```python
from build123d import *

# Parameters (mm, degrees)
SKETCH_1_R      = 1.35
SKETCH_1_R_2    = 1.3
EXTRUDE_1_DEPTH = 3


with BuildPart() as part:
    # 草图1 → 凸台-拉伸1 (new body)
    with BuildSketch(Plane.XY.offset(3)):
        with BuildLine():
            Line((291.111009591, 60.850346254), (291.08477602, 16.850708535))
            ThreePointArc((291.08477602, 16.850708535), (291.962190742, 14.728864681), (294.08298682, 13.848920402))
            Line((294.08298682, 13.848920402), (338.082927985, 13.82268665))
            ThreePointArc((338.082927985, 13.82268665), (340.20477184, 14.700101372), (341.084716119, 16.82089745))
            Line((341.084716119, 16.82089745), (341.11094969, 60.820535169))
            ThreePointArc((341.11094969, 60.820535169), (340.233534968, 62.942379024), (338.11273889, 63.822323303))
            Line((338.11273889, 63.822323303), (294.112797724, 63.848557054))
            ThreePointArc((294.112797724, 63.848557054), (291.990953869, 62.971142333), (291.111009591, 60.850346254))
        make_face()
        with Locations(Location((338.084716652, 16.822686117, 0), (0, 0, 180))):
            Circle(SKETCH_1_R, mode=Mode.SUBTRACT)
        with Locations(Location((294.111009057, 60.848557587, 0), (0, 0, 180))):
            Circle(SKETCH_1_R, mode=Mode.SUBTRACT)
        with Locations(Location((338.110950223, 60.822323836, 0), (0, 0, 180))):
            Circle(SKETCH_1_R, mode=Mode.SUBTRACT)
        with Locations(Location((294.084775487, 16.848919869, 0), (0, 0, 180))):
            Circle(SKETCH_1_R, mode=Mode.SUBTRACT)
        with Locations(Location((316.118760947, 29.316353397, 0), (0, 0, 180))):
            Circle(SKETCH_1_R_2, mode=Mode.SUBTRACT)
        with Locations(Location((316.098042718, 48.316807582, 0), (0, 0, 180))):
            Circle(SKETCH_1_R_2, mode=Mode.SUBTRACT)
        Polygon((304.601683778, 44.942477784), (327.602382744, 44.928764251), (327.595108581, 32.728346323), (304.594409616, 32.742059855), align=None, mode=Mode.SUBTRACT)
    extrude(amount=-EXTRUDE_1_DEPTH)


solid = part.part
```
Geometry: final body of the model. Coordinates: model frame, mm. Coordinates: 2 decimals unless noted, no trailing zeros. Write each loop counter-clockwise with the first axis right and the second up, starting at its lowest first coordinate (ties: lowest second). Pieces come first, ordered by that corner, then holes. Notation, with made-up numbers: M 81.25,15 L 92.25,15 A13 ccw 92.25,36 Z; hole C 12,38.25 d2. An arc over 180 degrees is marked long. Answer as CSV lines item,"result". Start each with the question number.
Q1. Cut plane B-B on y = 36.5. Return the cut outline in (x, z).
Q2. Cut plane A-A on x = 311. Return the cut outline in (y, z).
Q3. Line query: line 1 (Y direction, x = 318, z = 2); line 2 (X direction, y = 40, z = 2.1); line 3 (Y direction, x = 338, z = 2.2). Output: solid intervals per line, ascending. Write a range as from..to.
Q4. Pin query (flat end, axial travel): P1, Ø1, axis at y = 30, z = 2.5, coming from the -X side; P2, Ø1, axis at x = 330.5, z = 2, coming from the -Y side. Return the tip coordinate at first contact, or that it passes through.
Q5. Cut plane C-C on z = 1.9. Return the cut outline in (x, y), then the cut area to 3 significant figures.
Q6. Mould query, pull axis X, two halves, no side actions, for faces 1 (the cylindrical face through (317.418, 29.259, 1.521)), 2 (the cylindrical face through (292.8, 16.44, 1.52)), 3 (the flat face through (316, 50, 0)), 4 (the cylindrical face through (291.94, 14.75, 1.52)). Classes: released by +X, released by -X, zero draft, split by the parting line, or undercut.
Findings below:
1,outline,"M 291.1,0 L 304.6,0 L 304.6,3 L 291.1,3 Z; M 327.6,0 L 341.1,0 L 341.1,3 L 327.6,3 Z"
2,outline,"M 13.84,0 L 32.74,0 L 32.74,3 L 13.84,3 Z; M 44.94,0 L 63.84,0 L 63.84,3 L 44.94,3 Z"
3,line 1,"y = 13.83..32.73, 44.93..63.83"
3,line 2,"x = 291.1..304.6, 327.6..341.1"
3,line 3,"y = 13.82..15.48, 18.17..59.48, 62.17..63.82"
4,P1,"stops at x = 291.09"
4,P2,"stops at y = 13.83"
5,outline,"M 291.08,16.85 A3 ccw 294.08,13.85 L 338.08,13.82 A3 ccw 341.08,16.82 L 341.11,60.82 A3 ccw 338.11,63.82 L 294.11,63.85 A3 ccw 291.11,60.85 Z; hole C 294.08,16.85 d2.7; hole C 294.11,60.85 d2.7; hole M 304.59,32.74 L 327.6,32.73 L 327.6,44.93 L 304.6,44.94 Z; hole C 316.1,48.32 d2.6; hole C 316.12,29.32 d2.6; hole C 338.08,16.82 d2.7; hole C 338.11,60.82 d2.7"
5,area,"2,180 mm2"
6,face 1,"undercut"
6,face 2,"undercut"
6,face 3,"zero draft"
6,face 4,"released by -X"
